Geometry: final body of the model. Coordinates: model frame, mm. A direction names the side the tool comes from. Coordinates: 2 decimals unless noted, no trailing zeros. Loops run counter-clockwise (first coordinate to the right, second up) from the corner with the lowest first, then second, coordinate; pieces in that order, holes last. Notation, with made-up numbers: (89.25, 17.5) -> (145.25, 17.5) arc R4 cw to (145.25, 21.5) -> close; hole circle Ø10 at (20, 42). An arc over 180 degrees is marked (long way). One line per item, written item: value. Start each with the question number.
Item 1: Section query B-B on x = 1. Return loops of the section in (y, z).
Item 2: Contact query for flat-ended pins moving along their axis: pin 1 Ø5 at (x, z) = (-0.5, -4) entering from -Y; pin 2 Ø3 at (x, z) = (-0.5, -2) entering from +Y. Output: stop coordinate, or through.
Item 3: Ray query, probe 1 along Z at (x, y) = (5.5, -1.45); probe 2 along Y at (x, z) = (-0.25, -1); probe 3 along X at (y, z) = (-0.8, 36). Return the intervals inside material, ascending. Write a range as from..to.
Item 4: Section query A-A on z = -3. Return loops of the section in (x, y).
Item 5: Set-up query: faces 1 (the cylindrical face through (3.865, 0.949, -3.204)), 2 (the flat face through (0, -1.25, -3)), 3 (the cylindrical face through (-3.849, 0.965, -3.204)), 4 (the flat face through (0, 1.25, -3)). Return all of +Z, -Z, +X, -X, +Y, -Y with unobstructed straight access to the full face (end or side cutting, diameter ignored); none if empty.
Autodesk Inventor part; units mm, degrees
ref_plane "YZ Plane" through (0, 0, 0) normal (1, 0, 0) x (0, 1, 0)
ref_plane "XZ Plane" through (0, 0, 0) normal (0, 1, 0) x (-1, 0, 0)
ref_plane "XY Plane" through (0, 0, 0) normal (0, 0, 1) x (1, 0, 0)
sketch "Sketch1" plane through (0, 0, 0) normal (0, 0, 1) x (1, 0, 0)
  line L0 (-5.5, 1.75) -> (5.5, 1.75)
  line L1 (6.5, 0.75) -> (6.5, -0.75)
  line L2 (5.5, -1.75) -> (-5.5, -1.75)
  line L3 (-6.5, -0.75) -> (-6.5, 0.75)
  line L4 (0, 0) -> (0, 3.6789) construction
  line L5 (0, 0) -> (3.0794, 0) construction
  arc A0 (-5.5, 1.75) -> (-6.5, 0.75) centre (-5.5, 0.75) ccw
  arc A1 (-6.5, -0.75) -> (-5.5, -1.75) centre (-5.5, -0.75) ccw
  arc A2 (5.5, -1.75) -> (6.5, -0.75) centre (5.5, -0.75) ccw
  arc A3 (6.5, 0.75) -> (5.5, 1.75) centre (5.5, 0.75) ccw
  point P0 (-6.5, 1.75)
  point P1 (6.5, -1.75)
  point P2 (6.5, 1.75)
  dimension "d0" = 13
  dimension "d1" = 3.5
  dimension "d2" = 1
  dimension "d3" = 1
extrude "Extrusion1" add sketch "Sketch1" along normal blind 40
sketch "Sketch2" plane through (0, 0, 0) normal (0, 0, -1) x (-1, 0, 0)
  line L0 (-3.15, 1.25) -> (3.15, 1.25)
  line L1 (4.15, 0.25) -> (4.15, -0.25)
  line L2 (3.15, -1.25) -> (-3.15, -1.25)
  line L3 (-4.15, -0.25) -> (-4.15, 0.25)
  line L4 (0, 0) -> (0, 2.3167) construction
  line L5 (0, 0) -> (2.0938, 0) construction
  arc A0 (-3.15, 1.25) -> (-4.15, 0.25) centre (-3.15, 0.25) ccw
  arc A1 (-4.15, -0.25) -> (-3.15, -1.25) centre (-3.15, -0.25) ccw
  arc A2 (3.15, -1.25) -> (4.15, -0.25) centre (3.15, -0.25) ccw
  arc A3 (4.15, 0.25) -> (3.15, 1.25) centre (3.15, 0.25) ccw
  point P0 (4.15, -1.25)
  point P1 (4.15, 1.25)
  point P2 (-4.15, -1.25)
  dimension "d6" = 8.3
  dimension "d7" = 2.5
  dimension "d8" = 1
extrude "Extrusion2" add sketch "Sketch2" along normal blind 6.5
properties part number "3d_JacintoDevKit_Addon - USB Type-C"
Reply:
1. outline: (-1.75, 0) -> (-1.25, 0) -> (-1.25, -6.5) -> (1.25, -6.5) -> (1.25, 0) -> (1.75, 0) -> (1.75, 40) -> (-1.75, 40) -> close
2. pin 1: stops at y = -1.25
2. pin 2: stops at y = 1.25
3. probe 1: z = 0..40
3. probe 2: y = -1.25..1.25
3. probe 3: x = -6.5..6.5
4. outline: (-4.15, -0.25) arc R1 ccw to (-3.15, -1.25) -> (3.15, -1.25) arc R1 ccw to (4.15, -0.25) -> (4.15, 0.25) arc R1 ccw to (3.15, 1.25) -> (-3.15, 1.25) arc R1 ccw to (-4.15, 0.25) -> close
5. face 1: -Z, +X, +Y
5. face 2: -Z, +X, -X, -Y
5. face 3: -Z, -X, +Y
5. face 4: -Z, +X, -X, +Y
